Can you work these out from the model? Positions are in its coordinate system, mm. Face numbers are marked on the shaded views. A direction names the side the tool comes from. Coordinates: 2 decimals unless noted, no trailing zeros. Loops run counter-clockwise (first coordinate to the right, second up) from the corner with the lowest first, then second, coordinate; pieces in that order, holes last. Notation, with made-up numbers: (51, -20.5) -> (110, -20.5) arc R6 cw to (110, -9.5) -> close; hole circle Ø4 at (12, 7). An arc over 180 degrees is marked (long way). Put each result on its own line as item: value. Start each with the question number.
Item 1: If we section it at A-A on z = 6.55: Please give me the cut outline in (x, y), plus the area to 3 significant figures.
Item 2: We'd pull the mould along X, two halves only. Please class the marked faces 4 and 5: pulls with the +X half, pulls with the -X half, needs draft (parallel to the pull), parting line crosses it, or undercut.
Item 3: Will these pins go through, and if not, where does the flat tip stop? P1, Ø7.5, axis at x = 0, y = 0, coming from the -Z side; P2, Ø2, axis at x = 13, y = -8, coming from the +Z side; P3, Ø2, axis at y = 7.5, z = 1.5, coming from the -X side; P4, Ø1.5, axis at y = 8, z = 2, coming from the +X side.
Item 4: If we section it at B-B on y = 0: Please give me the cut outline in (x, z) (3 decimals), plus the area to 3 significant figures.
Item 5: If we section it at C-C on x = 0: Please give me the cut outline in (y, z), plus the area to 3 significant figures.
Item 6: For the marked faces 1, 2 and 3, which set-ups out of +Z, -Z, +X, -X, +Y, -Y let a thin tool reach every point of the face, with its end or its side?
Item 7: Please list where these lines run through material, in increasing order: L1, parallel to Z at x = -16.75, y = -3; L2, parallel to X at y = -1.75, z = 6.55; L3, parallel to X at y = 3.5, z = 10.75. Write a range as from..to.
Item 8: If we section it at D-D on z = 9.5: Please give me the cut outline in (x, y).
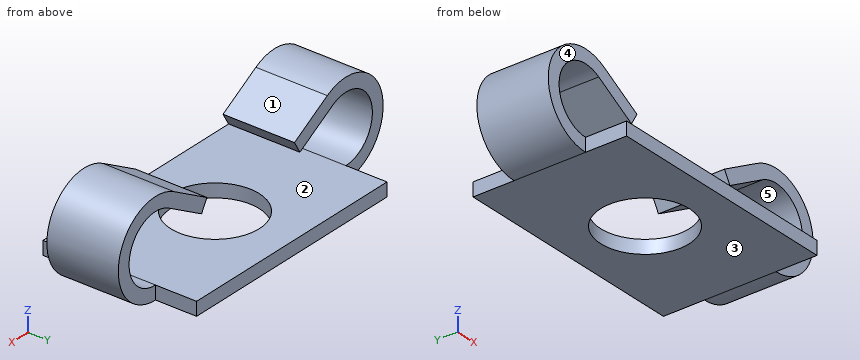
```python
from build123d import *

# Parameters (mm, degrees)
SKETCH_1_W      = 33.5
SKETCH_1_H      = 21.5
SKETCH_1_R      = 6.2
EXTRUDE_1_DEPTH = 1.9
EXTRUDE_2_DEPTH = 5


with BuildPart() as part:
    # Эскиз1 → Бобышка-Вытянуть1 (new body)
    with BuildSketch(Plane.XY):
        Rectangle(SKETCH_1_W, SKETCH_1_H)
        Circle(SKETCH_1_R, mode=Mode.SUBTRACT)
    extrude(amount=EXTRUDE_1_DEPTH)

    # Эскиз3 → Бобышка-Вытянуть2 (add, symmetric)
    with BuildSketch(Plane(origin=(0, 0, 0), x_dir=(1, 0, 0), z_dir=(0, 1, 0))):
        with BuildLine():
            Line((-14.425, -10.577018128), (-8.65, -7.242820323))
            Line((-8.65, -7.242820323), (-7.7, -8.88826859))
            Line((-7.7, -8.88826859), (-13.475, -12.222466395))
            ThreePointArc((-13.475, -12.222466395), (-23.076814162, -8.245264745), (-16.75, 0))
            Line((-16.75, 0), (-16.75, -1.9))
            ThreePointArc((-16.75, -1.9), (-21.241555092, -7.75350856), (-14.425, -10.577018128))
        make_face()
    extrude_2 = extrude(amount=EXTRUDE_2_DEPTH, both=True)

    # Зеркальное отражение1: Бобышка-Вытянуть2 across plane
    add(extrude_2.mirror(Plane(origin=(0, 0, 0), x_dir=(0, 0, 1), z_dir=(1, 0, 0))))


solid = part.part
```
Solutions:
1. outline: (-23.3, -5) -> (-21.4, -5) -> (-21.4, 5) -> (-23.3, 5) -> close; (21.4, -5) -> (23.3, -5) -> (23.3, 5) -> (21.4, 5) -> close
1. area: 38.0 mm^2
2. face 4: needs draft
2. face 5: undercut
3. P1: through
3. P2: z = 1.9
3. P3: x = -16.75
3. P4: x = 16.75
4. outline: (-16.75, 0) -> (-6.2, 0) -> (-6.2, 1.9) -> (-16.75, 1.9) arc R4.65 cw (long way) to (-14.425, 10.577) -> (-8.65, 7.243) -> (-7.7, 8.888) -> (-13.475, 12.222) arc R6.55 ccw (long way) to start; (6.2, 0) -> (16.75, 0) arc R6.55 ccw (long way) to (13.475, 12.222) -> (7.7, 8.888) -> (8.65, 7.243) -> (14.425, 10.577) arc R4.65 cw (long way) to (16.75, 1.9) -> (6.2, 1.9) -> close
4. area: 143 mm^2
5. outline: (-10.75, 0) -> (-6.2, 0) -> (-6.2, 1.9) -> (-10.75, 1.9) -> close; (6.2, 0) -> (10.75, 0) -> (10.75, 1.9) -> (6.2, 1.9) -> close
5. area: 17.3 mm^2
6. face 1: +Z, +Y, -Y
6. face 2: +Y, -Y
6. face 3: -Z, +X, -X, +Y, -Y
7. L1: 0..1.9, 11.2..13.1
7. L2: -23.3..-21.4, 21.4..23.3
7. L3: -21.78..-18.75, -14.75..-10.92, 10.92..14.75, 18.75..21.78
8. outline: (-22.6, -5) -> (-20.34, -5) -> (-20.34, 5) -> (-22.6, 5) -> close; (-12.56, -5) -> (-8.76, -5) -> (-8.76, 5) -> (-12.56, 5) -> close; (8.76, -5) -> (12.56, -5) -> (12.56, 5) -> (8.76, 5) -> close; (20.34, -5) -> (22.6, -5) -> (22.6, 5) -> (20.34, 5) -> close
